```python
from build123d import *

# Parameters (mm, degrees)
F0_W      = 101.6
F0_H      = 5.08
F1_DEPTH  = 25.4
F0_H_2    = 35
F2_DEPTH  = 5.08
F1_FACE_W = 25.4
F1_FACE_H = 45.1612
F3_DEPTH  = 5.08


with BuildPart() as f1:
    # F0 (on Front) → F1 (new body)
    with BuildSketch(Plane.XZ):
        Polygon((0, -5.08), (0, 0), (0, 35), (0, 40.08), (-5.08, 40.08), (-5.08, -5.0812), (0, -5.0812), align=None)
        with Locations((50.8, -2.54)):
            Rectangle(F0_W, F0_H)
        Polygon((101.6, 35), (101.6, 0), (101.6, -5.08), (101.6, -5.0812), (106.68, -5.0812), (106.68, 40.08), (101.6, 40.08), align=None)
        with Locations((50.8, 37.54)):
            Rectangle(F0_W, F0_H)
    extrude(amount=F1_DEPTH)

    # F0 (on Front) → F2 (join)
    with BuildSketch(Plane.XZ):
        with Locations((50.8, 17.5)):
            Rectangle(F0_W, F0_H_2)
    extrude(amount=F2_DEPTH)

    # F1_face (on face) → F3 (cut)
    with BuildSketch(Plane(origin=(-5.08, -12.7, 17.4994), x_dir=(0, -1, 0), z_dir=(-1, 0, 0))):
        Rectangle(F1_FACE_W, F1_FACE_H)
    extrude(amount=-F3_DEPTH, mode=Mode.SUBTRACT)


solid = f1.part
```
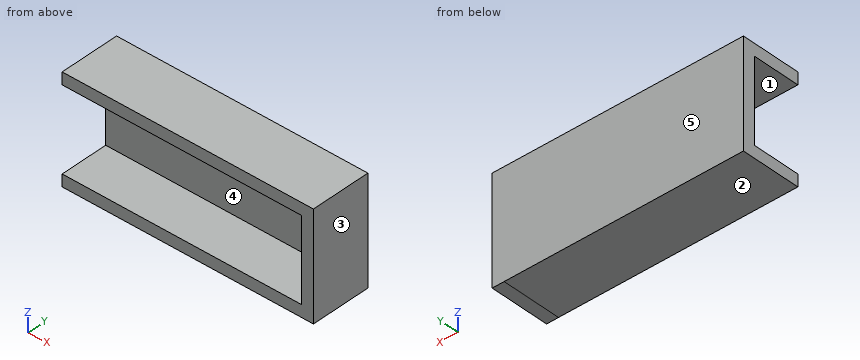
Work out the finished part from the listing and answer in its coordinate system (mm). Face numbers are marked on the shaded views. A direction names the side the tool comes from. Give positions to 0.01 mm unless a question says otherwise; leave off trailing zeros. Write each loop counter-clockwise with the first axis right and the second up, starting at its lowest first coordinate (ties: lowest second). Pieces come first, ordered by that corner, then holes. Notation, with made-up numbers: (-39, 33.5) -> (9, 33.5) arc R23 ccw to (9, 68.5) -> close; hole circle Ø4 at (14.25, 36). An arc over 180 degrees is marked (long way). Write item = value, one per line.
Q1. Consider line 1 along Z through (x, y) = (69, -10.5); line 2 along Z through (x, y) = (34.5, -4.75); line 3 along X through (y, z) = (-10, 33). Determine where each line is inside the solid, lowest interval first.
Computed values:
line_1 = -5.08 to 0, 35 to 40.08
line_2 = -5.08 to 40.08
line_3 = 101.6 to 106.68
Q2. Flat-ended cylindrical pins translate along their axes: pin 1 Ø6 at (y, z) = (-13, 24.5) entering from -X; pin 2 Ø8 at (x, z) = (82.5, 22.5) entering from -Y. Find the tip coordinate at first contact, or state that the pin passes through.
Computed values:
pin_1 = 101.6
pin_2 = -5.08
Q3. A tool of negligible diameter and unlimited length cuts with its end or side. For the marked faces 4 and 5, from which of +Z, -Z, +X, -X, +Y, -Y can it reach the whole face along a straight path? Write none if from no direction.
Computed values:
face_4 = -X, -Y
face_5 = +Z, -Z, +X, -X, +Y
Q4. For a pull along Z with two mould halves and no side action, classify the marked faces 1, 2 and 3 as pulls with the +Z half, pulls with the -Z half, needs draft (parallel to the pull), parting line crosses it, or undercut.
Computed values:
face_1 = undercut
face_2 = pulls with the -Z half
face_3 = needs draft
Q5. Section A-A on z = 9 is taken. Determine the outline of the cut face in (x, y).
Computed values:
outline = (0, -5.08) -> (101.6, -5.08) -> (101.6, -25.4) -> (106.68, -25.4) -> (106.68, 0) -> (0, 0) -> close
Q6. Section C-C on x = 13 is taken. Determine the outline of the cut face in (y, z), and give its area (3 significant figures).
Computed values:
outline = (-25.4, -5.08) -> (0, -5.08) -> (0, 40.08) -> (-25.4, 40.08) -> (-25.4, 35) -> (-5.08, 35) -> (-5.08, 0) -> (-25.4, 0) -> close
area = 436 mm^2
